Check sheet for the modelled part. Datum: model origin and axes. Units: mm. A direction names the side the tool comes from. Coordinates: 2 decimals unless noted, no trailing zeros. Loops run counter-clockwise (first coordinate to the right, second up) from the corner with the lowest first, then second, coordinate; pieces in that order, holes last.
```python
from build123d import *

# Parameters (mm, degrees)
F0_W          = 30.7596123494
F0_H          = 2
F1_DEPTH      = 2
F2_DEPTH      = 3
F2_DEPTH_BACK = 1
F4_DEPTH      = 2
F6_DEPTH      = 2


# Not quite as in the source:
# - a feature names something its author has since deleted; it is built from what else it names


with BuildPart() as f1:
    # F0 (on Top) → F1 (new body)
    with BuildSketch(Plane.XY):
        Polygon((40.7596123494, 2), (40.7596123494, 0), (90, 8.6824088833), (90, 10.6824088833), align=None)
        with Locations((25.3798061747, 1)):
            Rectangle(F0_W, F0_H)
    extrude(amount=F1_DEPTH)

    # F0 (on Top) → F2 (join, two sides)
    with BuildSketch(Plane.XY) as f2_sk:
        Polygon((0, 3), (0, 0), (10, 0), (10, 2), (10, 3), align=None)
    extrude(amount=F2_DEPTH)
    extrude(f2_sk.sketch, amount=-F2_DEPTH_BACK)

    # F3 (on face) → F4 (join)
    with BuildSketch(Plane.XZ):
        with BuildLine():
            ThreePointArc((1.75, 1), (3, -0.25), (4.25, 1))
            Line((4.25, 1), (1.75, 1))
        make_face()
        with BuildLine():
            Line((1.75, 1), (4.25, 1))
            ThreePointArc((4.25, 1), (3, 2.25), (1.75, 1))
        make_face()
        with BuildLine():
            ThreePointArc((8.25, 1), (7, 2.25), (5.75, 1))
            Line((5.75, 1), (8.25, 1))
        make_face()
        with BuildLine():
            Line((8.25, 1), (5.75, 1))
            ThreePointArc((5.75, 1), (7, -0.25), (8.25, 1))
        make_face()
    extrude(amount=F4_DEPTH)

    # F5 (on Top) → F6 (join)
    with BuildSketch(Plane.XY):
        Polygon((42, -20), (22, 0), (20, 0), (40, -20), align=None)
    extrude(amount=F6_DEPTH)


solid = f1.part
```
1) Set-up check for faces 1 (the cylindrical face through (8.25, -0.99, 0.95)), 2 (the flat face through (3, -2, 1)), 3 (the flat face through (32, -10, 1)), 4 (the flat face through (50, 2, 2)): record each of +Z, -Z, +X, -X, +Y, -Y from which the full face is reachable in a straight line by a thin tool's end or side.
Answer sheet:
face 1: -Y
face 2: +Z, -Z, -X, -Y
face 3: +Z, -Z, +X
face 4: +Z, +X, +Y, -Y
2) Scan lines: line 1 (Y direction, x = 8.5, z = 0.5); line 2 (Y direction, x = 30, z = 1.9); line 3 (Z direction, x = 30, y = -9.5). Record each from-to range of solid material in increasing order.
Answer sheet:
line 1: y = 0 to 3
line 2: y = -10 to -8, 0 to 2
line 3: z = 0 to 2
3) Section check B-B on z = 1. Enter the section's corners in (x, y).
Answer sheet:
outline: (0, 0) - (1.75, 0) - (1.75, -2) - (4.25, -2) - (4.25, 0) - (5.75, 0) - (5.75, -2) - (8.25, -2) - (8.25, 0) - (20, 0) - (40, -20) - (42, -20) - (22, 0) - (40.76, 0) - (90, 8.68) - (90, 10.68) - (40.76, 2) - (10, 2) - (10, 3) - (0, 3) - close
4) Section check D-D on y = -10. Enter the section's corners in (x, z).
Answer sheet:
outline: (30, 0) - (32, 0) - (32, 2) - (30, 2) - close
5) Section check C-C on x = 3. Enter the section's corners in (y, z).
Answer sheet:
outline: (-2, -0.25) - (0, -0.25) - (0, -1) - (3, -1) - (3, 3) - (0, 3) - (0, 2.25) - (-2, 2.25) - close
6) Mould release check, pull along Y, two halves, no side actions. Record for faces 5 (the flat face through (31, 0, 1)), 6 (the flat face through (0, 2, 1)), 7 (the flat face through (5, 3, 1)): +Y half, -Y half, draft (parallel to the pull), parting line (faces both ways), or undercut.
Answer sheet:
face 5: undercut
face 6: draft
face 7: +Y half
7) Depth check by flat-ended pin: pin 1 (2 mm diameter, centred on x = 5.5, z = 1, fed in from +Y); pin 2 (1.2 mm diameter, centred on x = 6.5, z = 1, fed in from -Y); pin 3 (2 mm diameter, centred on x = 27.5, z = 1.5, fed in from -Y). Enter the tip coordinate at first touch or a pass-through.
Answer sheet:
pin 1: stops at y = 3
pin 2: stops at y = -2
pin 3: stops at y = -8.5
8) Section check A-A on x = 25.5. Enter the section's corners in (y, z), plus the area to 3 significant figures.
Answer sheet:
outline: (-5.5, 0) - (-3.5, 0) - (-3.5, 2) - (-5.5, 2) - close; (0, 0) - (2, 0) - (2, 2) - (0, 2) - close
area: 8.00 mm2
